Work out the finished part from the listing and answer in its coordinate system (mm). Face numbers are marked on the shaded views. Round coordinates to 2 decimals unless told otherwise and drop trailing zeros. Write each loop counter-clockwise with the first axis right and the second up, starting at its lowest first coordinate (ties: lowest second). Pieces come first, ordered by that corner, then holes. Notation, with made-up numbers: M 44,51.5 L 80,51.5 A34 ccw 80,90.5 Z; hole C -37,-20.75 d10. An arc over 180 degrees is marked long. One line per item, written item: value. Start each with the question number.
Q1. Given pin 1 Ø1.5 at (x, y) = (-115.5, 22.5) entering from -Z; pin 2 Ø2.5 at (y, z) = (160.5, 2.5) entering from +X; pin 3 Ø1.5 at (y, z) = (148.5, 3) entering from -X; pin 4 Ø2.5 at (x, z) = (-16.5, 1.5) entering from +Y, each flat-ended and moving along its own axis, determine where each tip first touches the part or whether it passes through.
Q2. The mould has two halves that part along Z. Classify the marked faces 1 and 2: released by +Z, released by -Z, zero draft, split by the parting line, or undercut.
Q3. Find section B-B (z = 3.1). Count the separate pieces of the cut face and the enclosed holes in it, and give its area (3 significant figures).
Q4. Consider probe 1 along Y at (x, z) = (-67, 1.65); probe 2 along X at (y, z) = (-1, 3.2); probe 3 along X at (y, z) = (7, 1.7). Determine where each line is inside the solid, lowest interval first.
Q5. Find section A-A (y = -5). Write down the section's boundary in (x, z), and give its area (3 significant figures).
from build123d import *

# Parameters (mm, degrees)
SKETCH1_W           = 20
SKETCH1_H           = 5
SKETCH1_W_2         = 5
SKETCH1_H_2         = 20
SKETCH1_W_3         = 25
SKETCH1_W_4         = 30
BOSS_EXTRUDE1_DEPTH = 5


with BuildPart() as part:
    # Sketch1 → Boss-Extrude1 (new body)
    with BuildSketch(Plane.XY):
        with BuildLine():
            Line((-39.784412909, 125.453201578), (-39.784412909, 135.453201578))
            Line((-39.784412909, 135.453201578), (-44.784412909, 135.453201578))
            Line((-44.784412909, 135.453201578), (-44.784412909, 155.453201578))
            Line((-44.784412909, 155.453201578), (-39.784412909, 155.453201578))
            Line((-39.784412909, 155.453201578), (-39.784412909, 165.453201578))
            Line((-39.784412909, 165.453201578), (-59.784412909, 165.453201578))
            Line((-59.784412909, 165.453201578), (-59.784412909, 160.453201578))
            Line((-59.784412909, 160.453201578), (-79.784412909, 160.453201578))
            Line((-79.784412909, 160.453201578), (-79.784412909, 165.453201578))
            Line((-79.784412909, 165.453201578), (-99.784412909, 165.453201578))
            Line((-99.784412909, 165.453201578), (-99.784412909, 155.453201578))
            Line((-99.784412909, 155.453201578), (-94.784412909, 155.453201578))
            Line((-94.784412909, 155.453201578), (-94.784412909, 135.453201578))
            Line((-94.784412909, 135.453201578), (-99.784412909, 135.453201578))
            Line((-99.784412909, 135.453201578), (-99.784412909, 125.453201578))
            add(Edge.make_bspline(
                [(-204.784412909, 21.843580993), (-197.506230119, 23.701939803), (-175.474625692, 30.348491442), (-128.147146094, 54.275433129), (-102.183870773, 95.209842597), (-99.784412909, 125.453201578)],
                knots=[0.089716065, 0.089716065, 0.089716065, 0.089716065, 0.220283612, 0.4864068, 1, 1, 1, 1], degree=3))
            Line((-204.784412909, 21.843580993), (-204.784412909, -21.546798422))
            Line((-204.784412909, -21.546798422), (-209.784412909, -21.546798422))
            Line((-209.784412909, -21.546798422), (-209.784412909, 20.618388045))
            add(Edge.make_bspline(
                [(-219.784412909, 18.453201578), (-214.791132261, 19.441715958), (-209.784412909, 20.618388045)],
                knots=[0, 0, 0, 0.0598328, 0.0598328, 0.0598328], degree=2))
            Line((-219.784412909, 18.453201578), (-219.784412909, -61.546798422))
            Line((-219.784412909, -61.546798422), (-194.784412909, -61.546798422))
            Line((-194.784412909, -61.546798422), (-194.784412909, -66.546798422))
            Line((-194.784412909, -66.546798422), (-219.784412909, -66.546798422))
            Line((-219.784412909, -66.546798422), (-219.784412909, -74.546798422))
            Line((-219.784412909, -74.546798422), (80.215587091, -74.546798422))
            Line((80.215587091, -74.546798422), (80.215587091, -66.546798422))
            Line((80.215587091, -66.546798422), (55.215587091, -66.546798422))
            Line((55.215587091, -66.546798422), (55.215587091, -61.546798422))
            Line((55.215587091, -61.546798422), (80.215587091, -61.546798422))
            Line((80.215587091, -61.546798422), (80.215587091, 18.453201578))
            add(Edge.make_bspline(
                [(80.215587091, 18.453201578), (75.222306443, 19.441715958), (70.215587091, 20.618388045)],
                knots=[0, 0, 0, 0.0598328, 0.0598328, 0.0598328], degree=2))
            Line((70.215587091, 20.618388045), (70.215587091, -21.546798422))
            Line((70.215587091, -21.546798422), (65.215587091, -21.546798422))
            Line((65.215587091, -21.546798422), (65.215587091, 21.843580993))
            add(Edge.make_bspline(
                [(65.215587091, 21.843580993), (57.937404301, 23.701939803), (35.905799874, 30.348491442), (-11.421679724, 54.275433129), (-37.384955046, 95.209842597), (-39.784412909, 125.453201578)],
                knots=[0.089716065, 0.089716065, 0.089716065, 0.089716065, 0.220283612, 0.4864068, 1, 1, 1, 1], degree=3))
        make_face()
        with Locations((-69.784412909, 127.953201578)):
            Rectangle(SKETCH1_W, SKETCH1_H, mode=Mode.SUBTRACT)
        with Locations((-69.784412909, 55.453201578)):
            Rectangle(SKETCH1_W_2, SKETCH1_H_2, mode=Mode.SUBTRACT)
        with Locations((-69.784412909, 95.453201578)):
            Rectangle(SKETCH1_W_2, SKETCH1_H_2, mode=Mode.SUBTRACT)
        with Locations((22.715587091, -64.046798422)):
            Rectangle(SKETCH1_W_3, SKETCH1_H, mode=Mode.SUBTRACT)
        with Locations((-22.284412909, -64.046798422)):
            Rectangle(SKETCH1_W_3, SKETCH1_H, mode=Mode.SUBTRACT)
        with Locations((-69.784412909, -64.046798422)):
            Rectangle(SKETCH1_W_4, SKETCH1_H, mode=Mode.SUBTRACT)
        with Locations((-117.284412909, -64.046798422)):
            Rectangle(SKETCH1_W_3, SKETCH1_H, mode=Mode.SUBTRACT)
        with Locations((-162.284412909, -64.046798422)):
            Rectangle(SKETCH1_W_3, SKETCH1_H, mode=Mode.SUBTRACT)
        with Locations((-69.784412909, 15.453201578)):
            Rectangle(SKETCH1_W_2, SKETCH1_H_2, mode=Mode.SUBTRACT)
        with Locations((-69.784412909, -24.546798422)):
            Rectangle(SKETCH1_W_2, SKETCH1_H_2, mode=Mode.SUBTRACT)
    extrude(amount=BOSS_EXTRUDE1_DEPTH)


solid = part.part
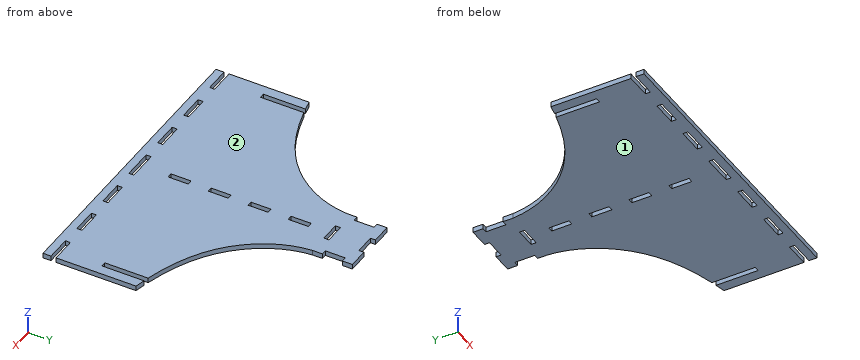
The answers:
1. pin 1: z = 0
1. pin 2: x = -39.78
1. pin 3: x = -94.78
1. pin 4: y = 70.85
2. face 1: released by -Z
2. face 2: released by +Z
3. separate pieces: 1
3. enclosed holes: 10
3. area: 41,400 mm2
4. probe 1: -74.55 to -66.55, -61.55 to 125.45, 130.45 to 160.45
4. probe 2: -219.78 to -209.78, -204.78 to 65.22, 70.22 to 80.22
4. probe 3: -219.78 to -209.78, -204.78 to -72.28, -67.28 to 65.22, 70.22 to 80.22
5. outline: M -219.78,0 L -209.78,0 L -209.78,5 L -219.78,5 Z; M -204.78,0 L 65.22,0 L 65.22,5 L -204.78,5 Z; M 70.22,0 L 80.22,0 L 80.22,5 L 70.22,5 Z
5. area: 1,450 mm2
